```python
from build123d import *

# Parameters (mm, degrees)
SKETCH1_R           = 2.15
BOSS_EXTRUDE1_DEPTH = 3
CUT_EXTRUDE1_REACH  = 5
CUT_EXTRUDE2_REACH  = 5
SKETCH5_R           = 1.6


with BuildPart() as part:
    # Sketch1 → Boss-Extrude1 (new body)
    with BuildSketch(Plane(origin=(0, 0, 0), x_dir=(1, 0, 0), z_dir=(0, 1, 0))):
        with BuildLine():
            Line((-43, 51), (43, 51))
            ThreePointArc((43, 51), (48.656854249, 48.656854249), (51, 43))
            Line((51, 43), (51, -66.5))
            ThreePointArc((51, -66.5), (48.656854249, -72.156854249), (43, -74.5))
            Line((43, -74.5), (-43, -74.5))
            ThreePointArc((-43, -74.5), (-48.656854249, -72.156854249), (-51, -66.5))
            Line((-51, -66.5), (-51, 43))
            ThreePointArc((-51, 43), (-48.656854249, 48.656854249), (-43, 51))
        make_face()
        with Locations((-31.5, 45)):
            Circle(SKETCH1_R, mode=Mode.SUBTRACT)
        with Locations((31.5, 45)):
            Circle(SKETCH1_R, mode=Mode.SUBTRACT)
        with Locations((-31.5, -70)):
            Circle(SKETCH1_R, mode=Mode.SUBTRACT)
        with Locations((31.5, -70)):
            Circle(SKETCH1_R, mode=Mode.SUBTRACT)
    extrude(amount=BOSS_EXTRUDE1_DEPTH)

    # Sketch3 → Cut-Extrude1 (cut, up to next)
    with BuildSketch(Plane(origin=(0, 3, 0), x_dir=(1, 0, 0), z_dir=(0, 1, 0)), mode=Mode.PRIVATE) as cut_extrude1_sk1:
        with BuildLine():
            Line((-24, -41), (24, -41))
            ThreePointArc((24, -41), (36.02081528, -36.02081528), (41, -24))
            Line((41, -24), (41, 24))
            ThreePointArc((41, 24), (36.02081528, 36.02081528), (24, 41))
            Line((24, 41), (-24, 41))
            ThreePointArc((-24, 41), (-36.02081528, 36.02081528), (-41, 24))
            Line((-41, 24), (-41, -24))
            ThreePointArc((-41, -24), (-36.02081528, -36.02081528), (-24, -41))
        make_face()
    cut_extrude1_tool1 = extrude(cut_extrude1_sk1.sketch, amount=-CUT_EXTRUDE1_REACH, mode=Mode.PRIVATE) & part.part
    add(cut_extrude1_tool1.solids().sort_by_distance((0, 3, 0))[0], mode=Mode.SUBTRACT)

    # Sketch5 → Cut-Extrude2 (cut, up to next)
    with BuildSketch(Plane(origin=(0, 3, 0), x_dir=(1, 0, 0), z_dir=(0, 1, 0)), mode=Mode.PRIVATE) as cut_extrude2_sk1:
        with Locations((21.612877951, -47.443396553)):
            Circle(SKETCH5_R)
    cut_extrude2_tool1 = extrude(cut_extrude2_sk1.sketch, amount=-CUT_EXTRUDE2_REACH, mode=Mode.PRIVATE) & part.part
    add(cut_extrude2_tool1.solids().sort_by_distance((21.612878, 3, 47.443397))[0], mode=Mode.SUBTRACT)
    # Sketch5 → Cut-Extrude2 (cut, up to next)
    with BuildSketch(Plane(origin=(0, 3, 0), x_dir=(1, 0, 0), z_dir=(0, 1, 0)), mode=Mode.PRIVATE) as cut_extrude2_sk2:
        with Locations((3.957960008, -64.39137202)):
            Circle(SKETCH5_R)
    cut_extrude2_tool2 = extrude(cut_extrude2_sk2.sketch, amount=-CUT_EXTRUDE2_REACH, mode=Mode.PRIVATE) & part.part
    add(cut_extrude2_tool2.solids().sort_by_distance((3.95796, 3, 64.391372))[0], mode=Mode.SUBTRACT)


solid = part.part
```
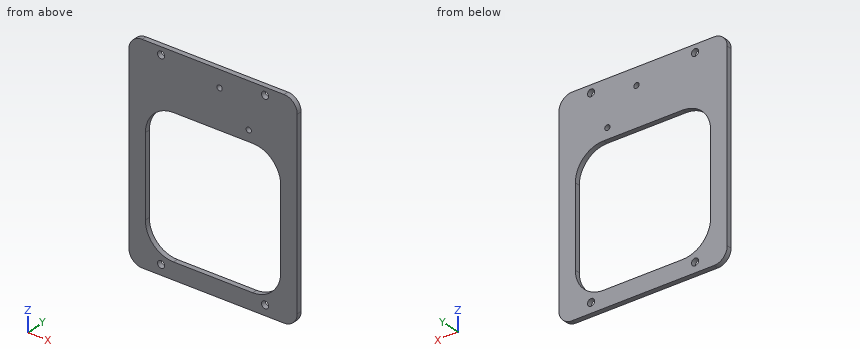
Model file for the job. Use its own axes, mm. Coordinates: 2 decimals unless noted, no trailing zeros. Loops run counter-clockwise (first coordinate to the right, second up) from the corner with the lowest first, then second, coordinate; pieces in that order, holes last. Notation, with made-up numbers: (44, 82) -> (87, 82) arc R6 ccw to (87, 93) -> close; hole circle Ø6 at (-17, 51.25). An arc over 180 degrees is marked (long way). Answer as a JSON object with one key per item and string values.
Q1. Probe probe 1 along X at (y, z) = (1.1, -23.5); probe 2 along Z at (x, y) = (-20, 0.9); probe 3 along Z at (x, y) = (-31.5, 2.3). List the from-to ranges inside material, lowest first.
Report:
{"probe 1": "x = -51 to -41, 41 to 51", "probe 2": "z = -51 to -41, 41 to 74.5", "probe 3": "z = -51 to -47.15, -42.85 to -39.26, 39.26 to 67.85, 72.15 to 74.5"}
Q2. Cut at B-B (x = 31.5). List the corners of the cut face in (y, z), and give its area (3 significant figures).
Report:
{"outline": "(0, -51) -> (3, -51) -> (3, -47.15) -> (0, -47.15) -> close; (0, -42.85) -> (3, -42.85) -> (3, -39.26) -> (0, -39.26) -> close; (0, 39.26) -> (3, 39.26) -> (3, 67.85) -> (0, 67.85) -> close; (0, 72.15) -> (3, 72.15) -> (3, 74.5) -> (0, 74.5) -> close", "area": "115 mm2"}
Q3. Cut at A-A (z = 0). List the corners of the cut face in (x, y).
Report:
{"outline": "(-51, 0) -> (-41, 0) -> (-41, 3) -> (-51, 3) -> close; (41, 0) -> (51, 0) -> (51, 3) -> (41, 3) -> close"}
Q4. Cut at D-D (y = 1.45). List the corners of the cut face in (x, z), and give its area (3 significant figures).
Report:
{"outline": "(-51, -43) arc R8 ccw to (-43, -51) -> (43, -51) arc R8 ccw to (51, -43) -> (51, 66.5) arc R8 ccw to (43, 74.5) -> (-43, 74.5) arc R8 ccw to (-51, 66.5) -> close; hole (-41, -24) arc R17 ccw to (-24, -41) -> (24, -41) arc R17 ccw to (41, -24) -> (41, 24) arc R17 ccw to (24, 41) -> (-24, 41) arc R17 ccw to (-41, 24) -> close; hole circle Ø4.3 at (-31.5, -45); hole circle Ø4.3 at (-31.5, 70); hole circle Ø3.2 at (3.96, 64.39); hole circle Ø3.2 at (21.61, 47.44); hole circle Ø4.3 at (31.5, -45); hole circle Ø4.3 at (31.5, 70)", "area": "6,200 mm2"}
Q5. Cut at C-C (z = 70). List the corners of the cut face in (x, y).
Report:
{"outline": "(-50.19, 0) -> (-33.65, 0) -> (-33.65, 3) -> (-50.19, 3) -> close; (-29.35, 0) -> (29.35, 0) -> (29.35, 3) -> (-29.35, 3) -> close; (33.65, 0) -> (50.19, 0) -> (50.19, 3) -> (33.65, 3) -> close"}
